The model under review builds one solid part; all positions refer to its coordinate system, in mm. Face numbers are marked on the shaded views. A direction names the side the tool comes from. Coordinates: 2 decimals unless noted, no trailing zeros. Write each loop counter-clockwise with the first axis right and the second up, starting at its lowest first coordinate (ties: lowest second). Pieces come first, ordered by that corner, then holes.
```python
from build123d import *

# Parameters (mm, degrees)
SKETCH1_W           = 3
SKETCH1_H           = 3
BOSS_EXTRUDE1_DEPTH = 2
SKETCH2_W           = 5
SKETCH2_H           = 5
BOSS_EXTRUDE2_DEPTH = 2
BOSS_EXTRUDE3_DEPTH = 2
BOSS_EXTRUDE4_DEPTH = 2


with BuildPart() as part:
    # Sketch1 → Boss-Extrude1 (new body)
    with BuildSketch(Plane(origin=(0, 0, 0), x_dir=(0, 0, -1), z_dir=(1, 0, 0))):
        Rectangle(SKETCH1_W, SKETCH1_H)
    extrude(amount=BOSS_EXTRUDE1_DEPTH)

    # Sketch2 → Boss-Extrude2 (add)
    with BuildSketch(Plane.ZY):
        Rectangle(SKETCH2_W, SKETCH2_H)
    extrude(amount=BOSS_EXTRUDE2_DEPTH)

    # Sketch4 → Boss-Extrude3 (add)
    with BuildSketch(Plane.XY.offset(2.5)):
        Polygon((-2, -2.5), (-4, -2.5), (-4, 1.5), (-2, 0.5), align=None)
    extrude(amount=-BOSS_EXTRUDE3_DEPTH)

    # Sketch5 → Boss-Extrude4 (add)
    with BuildSketch(Plane(origin=(0, 0, -2.5), x_dir=(-1, 0, 0), z_dir=(0, 0, -1))):
        Polygon((2, 2.5), (2, 0.5), (4, 1.5), (4, 2.5), align=None)
    extrude(amount=-BOSS_EXTRUDE4_DEPTH)


solid = part.part
```
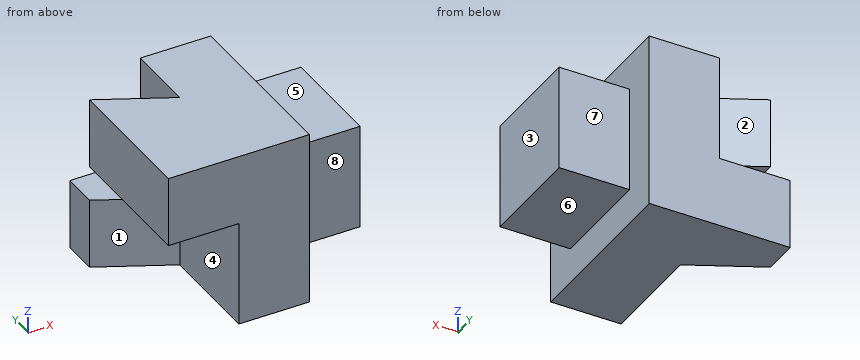
Item 1: Machinability: for the marked faces 5, 6, 7 and 8, which of the approach directions +Z, -Z, +X, -X, +Y, -Y give a long, thin tool a straight path to every point of the face, cutting with its end or side? Answer none if there is none.
Solved:
face 5: +Z, +X, +Y, -Y
face 6: -Z, +X, +Y, -Y
face 7: +Z, -Z, +X, +Y
face 8: +Z, -Z, +X, -Y
Item 2: Take a section at D-D, the plane x = -2.85. Write out the cut boundary in (y, z) (3 decimals).
Solved:
outline: (-2.5, 0.5) - (0.925, 0.5) - (0.925, 2.5) - (-2.5, 2.5) - close; (0.925, -2.5) - (2.5, -2.5) - (2.5, -0.5) - (0.925, -0.5) - close
Item 3: Mouldability with a two-part tool opening along X and no side actions: class the marked faces 1, 2, 3 and 4 as pulls with the +X half, pulls with the -X half, needs draft (parallel to the pull), parting line crosses it, or undercut.
Solved:
face 1: pulls with the -X half
face 2: undercut
face 3: pulls with the +X half
face 4: undercut
Item 4: To check wall thickness, follow line 1 along X through (y, z) = (0.1, -0.85); line 2 along X through (y, z) = (0.1, 2.25); line 3 along Z through (x, y) = (-3.75, 0.25). State the ranges of each line that lie inside material, in increasing order.
Solved:
line 1: x = -2 to 2
line 2: x = -4 to 0
line 3: z = 0.5 to 2.5
Item 5: Take a section at C-C, the plane y = -0.75. Write out the cut boundary in (x, z).
Solved:
outline: (-4, 0.5) - (-2, 0.5) - (-2, -2.5) - (0, -2.5) - (0, -1.5) - (2, -1.5) - (2, 1.5) - (0, 1.5) - (0, 2.5) - (-4, 2.5) - close
Item 6: For pin 1 (2 mm diameter, centred on x = 0.5, z = -0.5, fed in from -Y); pin 2 (0.6 mm diameter, centred on x = -3, y = -1, fed in from -Z); pin 3 (0.6 mm diameter, centred on x = 0.5, z = 0.5, fed in from +Y); pin 4 (1.6 mm diameter, centred on x = 1, y = 0.5, fed in from +Z), all flat-tipped, find the tip position at first contact; note any pin that passes through.
Solved:
pin 1: stops at y = -2.5
pin 2: stops at z = 0.5
pin 3: stops at y = 1.5
pin 4: stops at z = 1.5
Item 7: Take a section at B-B, the plane z = 0.8. Write out the cut boundary in (x, y), plus the area to 3 significant figures.
Solved:
outline: (-4, -2.5) - (0, -2.5) - (0, -1.5) - (2, -1.5) - (2, 1.5) - (0, 1.5) - (0, 2.5) - (-2, 2.5) - (-2, 0.5) - (-4, 1.5) - close
area: 23.0 mm2
Item 8: Take a section at A-A, the plane y = 0.65. Write out the cut boundary in (x, z), plus the area to 3 significant figures.
Solved:
outline: (-4, 0.5) - (-2.3, 0.5) - (-2.3, 2.5) - (-4, 2.5) - close; (-2.3, -2.5) - (0, -2.5) - (0, -1.5) - (2, -1.5) - (2, 1.5) - (0, 1.5) - (0, 2.5) - (-2, 2.5) - (-2, -0.5) - (-2.3, -0.5) - close
area: 20.0 mm2
